Work out the finished part from the listing and answer in its coordinate system (mm). A direction names the side the tool comes from. Coordinates: 2 decimals unless noted, no trailing zeros. Loops run counter-clockwise (first coordinate to the right, second up) from the corner with the lowest first, then second, coordinate; pieces in that order, holes last. Notation, with made-up numbers: (-17, 21) - (3, 21) arc R9 cw to (3, 29) - close; hole circle Ø11 at (-23.75, 6). An arc over 180 degrees is marked (long way). Write each question's results on one line, items separated by ' | '. Start each with the question number.
Item 1: A tool of negligible diameter and unlimited length cuts with its end or side. For faces 4 (the face through (16.5, 1.2, -1.9)), 5 (the face through (6.5, 1, -2)), 6 (the face through (4.75, 1, -4)), from which of +Z, -Z, +X, -X, +Y, -Y can it reach the whole face along a straight path? Write none if from no direction.
Item 2: Section A-A, the plane y = 1.2 is taken. Write down the section's boundary in (x, z).
Item 3: Consider probe 1 along X at (y, z) = (1.4, -2); probe 2 along Z at (x, y) = (13.5, 1.6); probe 3 along X at (y, z) = (1, -4.6). Determine where each line is inside the solid, lowest interval first. Write a range as [from, to].
Item 4: Section B-B, the plane z = -2 is taken. Write down the section's boundary in (x, y), plus the area to 3 significant figures.
Item 5: Section C-C, the plane x = 1.25 is taken. Write down the section's boundary in (y, z).
Item 6: Each of these flat-tipped pins is pushed along its axis until it touches: pin 1 Ø1.5 at (y, z) = (1.5, 0) entering from +X; pin 2 Ø1.2 at (y, z) = (1, -4.5) entering from -X; pin 3 Ø2 at (x, z) = (13.5, -2) entering from -Y. Where does it stop, or does it pass through?
Item 7: Section D-D, the plane z = -4.1 is taken. Write down the section's boundary in (x, y).
Item 8: For a pull along X with two mould halves and no side action, classify faces 1 (the face through (6, 1, -3.452)), 2 (the face through (-9.5, 1.2, -2.1)), 3 (the face through (3, 1, 1)) as +X half, -X half, draft (parallel to the pull), parting line (faces both ways), or undercut.
from build123d import *

# Parameters (mm, degrees)
SKETCH1_R           = 3
SKETCH1_R_2         = 1.75
BOSS_EXTRUDE1_DEPTH = 2.5


with BuildPart() as part:
    # Sketch1 → Boss-Extrude1 (new body)
    with BuildSketch(Plane(origin=(0, 0, 0), x_dir=(1, 0, 0), z_dir=(0, 1, 0))):
        with Locations((-6.5, 2)):
            Circle(SKETCH1_R)
        with Locations((-6.5, 2)):
            Circle(SKETCH1_R_2, mode=Mode.SUBTRACT)
        with BuildLine():
            Line((7, 0), (0, 0))
            Line((0, 0), (0, 4))
            Line((0, 4), (2.25, 4))
            Line((2.25, 4), (2.25, 5))
            Line((2.25, 5), (-6.5, 5))
            ThreePointArc((-6.5, 5), (-4.378679656, 4.121320344), (-3.5, 2))
            ThreePointArc((-3.5, 2), (-4.378679656, -0.121320344), (-6.5, -1))
            Line((-6.5, -1), (13.5, -1))
            ThreePointArc((13.5, -1), (10.5, 2), (13.5, 5))
            Line((13.5, 5), (4.75, 5))
            Line((4.75, 5), (4.75, 4))
            Line((4.75, 4), (7, 4))
            Line((7, 4), (7, 0))
        make_face()
        Polygon((2.25, 4), (0, 4), (0, 0), (7, 0), (7, 4), (4.75, 4), (4.75, 3.451807229), (6.5, 3.451807229), (6.5, 0.55), (0.5, 0.55), (0.5, 3.451807229), (2.25, 3.451807229), align=None)
        with Locations((13.5, 2)):
            Circle(SKETCH1_R)
        with Locations((13.5, 2)):
            Circle(SKETCH1_R_2, mode=Mode.SUBTRACT)
    extrude(amount=BOSS_EXTRUDE1_DEPTH)


solid = part.part
Answer key:
1) face 4: +X, +Y, -Y | face 5: +Y, -Y | face 6: -Z, +Y, -Y
2) outline: (-6.5, -5) - (2.25, -5) - (2.25, -3.45) - (0.5, -3.45) - (0.5, -0.55) - (6.5, -0.55) - (6.5, -3.45) - (4.75, -3.45) - (4.75, -5) - (13.5, -5) arc R3 ccw to (13.5, 1) - (-6.5, 1) arc R3 ccw to start; hole circle Ø3.5 at (-6.5, -2); hole circle Ø3.5 at (13.5, -2)
3) probe 1: x = [-9.5, -8.25], [-4.75, 0.5], [6.5, 11.75], [15.25, 16.5] | probe 2: z = [-5, -3.75], [-0.25, 1] | probe 3: x = [-8, 2.25], [4.75, 15]
4) outline: (-9.5, 0) - (-8.25, 0) - (-8.25, 2.5) - (-9.5, 2.5) - close; (-4.75, 0) - (0.5, 0) - (0.5, 2.5) - (-4.75, 2.5) - close; (6.5, 0) - (11.75, 0) - (11.75, 2.5) - (6.5, 2.5) - close; (15.25, 0) - (16.5, 0) - (16.5, 2.5) - (15.25, 2.5) - close | area: 32.5 mm^2
5) outline: (0, -5) - (2.5, -5) - (2.5, -3.45) - (0, -3.45) - close; (0, -0.55) - (2.5, -0.55) - (2.5, 1) - (0, 1) - close
6) pin 1: stops at x = 16.23 | pin 2: stops at x = -8.82 | pin 3: passes through
7) outline: (-8.64, 0) - (2.25, 0) - (2.25, 2.5) - (-8.64, 2.5) - close; (4.75, 0) - (15.64, 0) - (15.64, 2.5) - (4.75, 2.5) - close
8) face 1: undercut | face 2: -X half | face 3: draft
